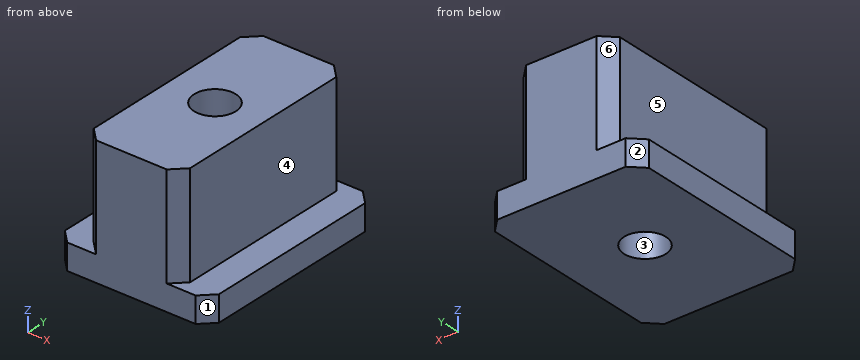
Autodesk Inventor part; units mm, degrees
ref_plane "YZ Plane" through (0, 0, 0) normal (1, 0, 0) x (0, 1, 0)
ref_plane "XZ Plane" through (0, 0, 0) normal (0, 1, 0) x (-1, 0, 0)
ref_plane "XY Plane" through (0, 0, 0) normal (0, 0, 1) x (1, 0, 0)
sketch "Esboço1" plane through (0, 0, 0) normal (0, 0, 1) x (1, 0, 0)
  line L0 (-6, 8) -> (6, 8)
  line L1 (6, 8) -> (6, -8)
  line L2 (6, -8) -> (-6, -8)
  line L3 (-6, -8) -> (-6, 8)
  line L4 (-6, 8) -> (6, -8) construction
  line L5 (6, 8) -> (-6, -8) construction
  point P0 (0, 0)
  dimension "d0" = 12
  dimension "d1" = 16
extrude "Extrusão1" add sketch "Esboço1" along normal blind 10
sketch "Esboço3" plane through (0, 0, 10) normal (0, 0, 1) x (1, 0, 0)
  line L0 (6, -8) -> (-6, -8)
  line L1 (-6, -8) -> (-6, 8)
  line L2 (-6, 8) -> (6, 8)
  line L3 (6, 8) -> (6, -8)
  line L4 (6, -8) -> (-6, 8) construction
  line L5 (-6, -8) -> (6, 8) construction
  line L6 (3.75, -8) -> (-3.75, -8)
  line L7 (-3.75, -8) -> (-3.75, 8)
  line L8 (-3.75, 8) -> (3.75, 8)
  line L9 (3.75, 8) -> (3.75, -8)
  line L10 (3.75, -8) -> (-3.75, 8) construction
  line L11 (-3.75, -8) -> (3.75, 8) construction
  point P0 (0, 0)
  dimension "d4" = 12
  dimension "d5" = 16
  dimension "d6" = 7.5
extrude "Extrusão2" cut sketch "Esboço3" against normal blind 8 contours L0 L9 L2 L3 | L0 L1 L2 L7
chamfer "Chanfro1" distance 1 angle 45 8 edges at (6, -8, 1) (-6, -8, 1) (6, 8, 1) (-6, 8, 1) (-3.75, -8, 6) (-3.75, 8, 6) (3.75, 8, 6) (3.75, -8, 6)
sketch "Esboço4" plane through (0, 0, 10) normal (0, 0, 1) x (1, 0, 0)
  circle A0 centre (0, 0) radius 1.5 construction
  dimension "d12" = 3
hole "Furo1" at (0, 0, 10) direction (0, 0, -1) diameter 3.242 end through all
properties part number "porcaDeslizante"
Could you check a few things on this model? Use its own coordinates, in mm. Face numbers are marked on the shaded views. A direction names the side the tool comes from. Round coordinates to 2 decimals unless told otherwise and drop trailing zeros. Order: outer loops, then holes, each group sorted by start corner. A loop starts at its lowest first (then second) coordinate and runs counter-clockwise, first axis right, second up.
(1) I'm going to push flat-ended pins straight in: pin 1 (1.5 mm diameter, centred on y = -3, z = 3, fed in from -X); pin 2 (1 mm diameter, centred on y = -1, z = 5, fed in from +X). Where does each tip first touch, or does it pass through?
Response values:
pin 1: stops at x = -3.75
pin 2: stops at x = 3.75
(2) Please list where these lines run through material, in increasing order: line 1 along X through (y, z) = (0, 6.25); line 2 along Y through (x, z) = (0, 7); line 3 along Z through (x, y) = (-4, -6).
Response values:
line 1: x = -3.75 to -1.62, 1.62 to 3.75
line 2: y = -8 to -1.62, 1.62 to 8
line 3: z = 0 to 2
(3) Imagine slicing it at C-C (y = 0). Write out the boundary of the cut face in (x, z).
Response values:
outline: (-6, 0) - (-1.62, 0) - (-1.62, 10) - (-3.75, 10) - (-3.75, 2) - (-6, 2) - close; (1.62, 0) - (6, 0) - (6, 2) - (3.75, 2) - (3.75, 10) - (1.62, 10) - close
(4) If we mould it in two halves opening along X, with no side actions, what happens to the marked faces 1, 2 and 3? For each: released by +X, released by -X, zero draft, split by the parting line, or undercut.
Response values:
face 1: released by +X
face 2: released by -X
face 3: undercut
(5) Imagine slicing it at A-A (x = 0). Write out the boundary of the cut face in (y, z).
Response values:
outline: (-8, 0) - (-1.62, 0) - (-1.62, 10) - (-8, 10) - close; (1.62, 0) - (8, 0) - (8, 10) - (1.62, 10) - close
(6) Imagine slicing it at D-D (x = 3.5). Write out the boundary of the cut face in (y, z), plus the area to 3 significant figures.
Response values:
outline: (-8, 0) - (8, 0) - (8, 2) - (7.25, 2) - (7.25, 10) - (-7.25, 10) - (-7.25, 2) - (-8, 2) - close
area: 148 mm2
(7) Which directions (+Z, -Z, +X, -X, +Y, -Y) give clear straight access to the entire face, cutting with the end or side of a thin tool? Please do the marked faces 4, 5 and 6.
Response values:
face 4: +Z, +X, +Y, -Y
face 5: +Z, -X, +Y, -Y
face 6: +Z, -X, +Y
(8) Imagine slicing it at B-B (z = 2.75). Write out the boundary of the cut face in (x, y), plus the area to 3 significant figures.
Response values:
outline: (-3.75, -7) - (-2.75, -8) - (2.75, -8) - (3.75, -7) - (3.75, 7) - (2.75, 8) - (-2.75, 8) - (-3.75, 7) - close; hole circle Ø3.24 at (0, 0)
area: 110 mm2
